The model under review builds one solid part; all positions refer to its coordinate system, in mm. Coordinates: 2 decimals unless noted, no trailing zeros. Write each loop counter-clockwise with the first axis right and the second up, starting at its lowest first coordinate (ties: lowest second). Pieces come first, ordered by that corner, then holes. Notation, with made-up numbers: (16, -11.5) - (47, -11.5) arc R33 ccw to (47, 21.5) - close; hole circle Ø3 at (58, -6). An arc over 180 degrees is marked (long way). Return JSON: item names as keys, results as strings. Group by question number.
(1) We need section B-B on x = 5.5. State the section outline as (y, z) points, then the cut area to 3 significant figures.
(2) We need section A-A on y = -37.5. State the section outline as (x, z) points, then the cut area to 3 significant figures.
(3) For pin 1 Ø6.5 at (x, y) = (-159, -94.5) entering from -Z; pin 2 Ø1.8 at (x, y) = (124, -21) entering from +Z; pin 3 Ø7.5 at (x, z) = (-165, 42.5) entering from +Y, all flat-tipped, find the tip position at first contact; note any pin that passes through.
(4) To check wall thickness, follow L1, parallel to Z at x = -309, y = -73; L2, parallel to Y at x = 258, z = 210; L3, parallel to Y at x = 310.5, z = -38.5. State the ranges of each line that lie inside material, in increasing order. Write a range as from..to.
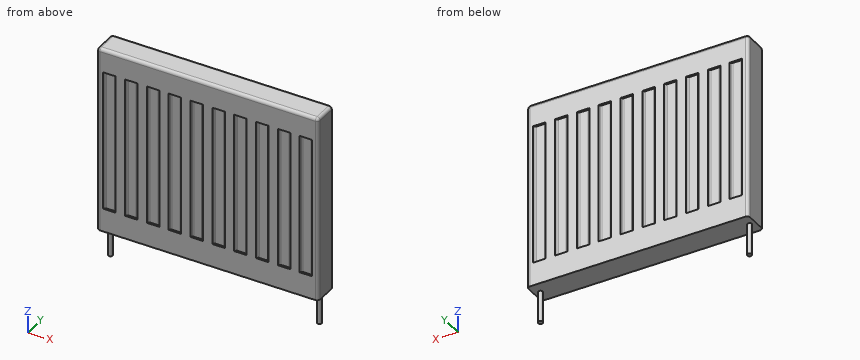
```python
from build123d import *

# Parameters (mm, degrees)
F0_W     = 710
F0_H     = 80
F1_DEPTH = 300
F2_R     = 7.5
F3_DEPTH = 100
F5_DEPTH = 225
F6_R     = 10


with BuildPart() as f1:
    # F0 (on Top) → F1 (new body, symmetric)
    with BuildSketch(Plane.XY):
        with Locations((9.33931, -58.683639)):
            Rectangle(F0_W, F0_H)
    extrude(amount=F1_DEPTH, both=True)

    # F2 (on face) → F3 (join)
    with BuildSketch(Plane(origin=(0, 0, -300), x_dir=(1, 0, 0), z_dir=(0, 0, -1))):
        with Locations((344.33931, 58.683639)):
            Circle(F2_R)
        with Locations((-325.66069, 58.683639)):
            Circle(F2_R)
    extrude(amount=F3_DEPTH)

    # F4 (on Top) → F5 (cut, symmetric)
    with BuildSketch(Plane.XY):
        with BuildLine():
            Line((-285.66069, -18.683639), (-325.66069, -18.683639))
            Line((-325.66069, -18.683639), (-322.124776, -22.897577))
            ThreePointArc((-322.124776, -22.897577), (-320.407645, -24.215178), (-318.294554, -24.683639))
            Line((-318.294554, -24.683639), (-293.026826, -24.683639))
            ThreePointArc((-293.026826, -24.683639), (-290.913735, -24.215178), (-289.196604, -22.897577))
            Line((-289.196604, -22.897577), (-285.66069, -18.683639))
        make_face()
        with BuildLine():
            Line((-215.66069, -18.683639), (-255.66069, -18.683639))
            Line((-255.66069, -18.683639), (-252.124776, -22.897577))
            ThreePointArc((-252.124776, -22.897577), (-250.407645, -24.215178), (-248.294554, -24.683639))
            Line((-248.294554, -24.683639), (-223.026826, -24.683639))
            ThreePointArc((-223.026826, -24.683639), (-220.913735, -24.215178), (-219.196604, -22.897577))
            Line((-219.196604, -22.897577), (-215.66069, -18.683639))
        make_face()
        with BuildLine():
            Line((-145.66069, -18.683639), (-185.66069, -18.683639))
            Line((-185.66069, -18.683639), (-182.124776, -22.897577))
            ThreePointArc((-182.124776, -22.897577), (-180.407645, -24.215178), (-178.294554, -24.683639))
            Line((-178.294554, -24.683639), (-153.026826, -24.683639))
            ThreePointArc((-153.026826, -24.683639), (-150.913735, -24.215178), (-149.196604, -22.897577))
            Line((-149.196604, -22.897577), (-145.66069, -18.683639))
        make_face()
        with BuildLine():
            Line((-75.66069, -18.683639), (-115.66069, -18.683639))
            Line((-115.66069, -18.683639), (-112.124776, -22.897577))
            ThreePointArc((-112.124776, -22.897577), (-110.407645, -24.215178), (-108.294554, -24.683639))
            Line((-108.294554, -24.683639), (-83.026826, -24.683639))
            ThreePointArc((-83.026826, -24.683639), (-80.913735, -24.215178), (-79.196604, -22.897577))
            Line((-79.196604, -22.897577), (-75.66069, -18.683639))
        make_face()
        with BuildLine():
            Line((-5.66069, -18.683639), (-45.66069, -18.683639))
            Line((-45.66069, -18.683639), (-42.124776, -22.897577))
            ThreePointArc((-42.124776, -22.897577), (-40.407645, -24.215178), (-38.294554, -24.683639))
            Line((-38.294554, -24.683639), (-13.026826, -24.683639))
            ThreePointArc((-13.026826, -24.683639), (-10.913735, -24.215178), (-9.196604, -22.897577))
            Line((-9.196604, -22.897577), (-5.66069, -18.683639))
        make_face()
        with BuildLine():
            Line((64.33931, -18.683639), (24.33931, -18.683639))
            Line((24.33931, -18.683639), (27.875224, -22.897577))
            ThreePointArc((27.875224, -22.897577), (29.592355, -24.215178), (31.705446, -24.683639))
            Line((31.705446, -24.683639), (56.973174, -24.683639))
            ThreePointArc((56.973174, -24.683639), (59.086265, -24.215178), (60.803396, -22.897577))
            Line((60.803396, -22.897577), (64.33931, -18.683639))
        make_face()
        with BuildLine():
            Line((134.33931, -18.683639), (94.33931, -18.683639))
            Line((94.33931, -18.683639), (97.875224, -22.897577))
            ThreePointArc((97.875224, -22.897577), (99.592355, -24.215178), (101.705446, -24.683639))
            Line((101.705446, -24.683639), (126.973174, -24.683639))
            ThreePointArc((126.973174, -24.683639), (129.086265, -24.215178), (130.803396, -22.897577))
            Line((130.803396, -22.897577), (134.33931, -18.683639))
        make_face()
        with BuildLine():
            Line((204.33931, -18.683639), (164.33931, -18.683639))
            Line((164.33931, -18.683639), (167.875224, -22.897577))
            ThreePointArc((167.875224, -22.897577), (169.592355, -24.215178), (171.705446, -24.683639))
            Line((171.705446, -24.683639), (196.973174, -24.683639))
            ThreePointArc((196.973174, -24.683639), (199.086265, -24.215178), (200.803396, -22.897577))
            Line((200.803396, -22.897577), (204.33931, -18.683639))
        make_face()
        with BuildLine():
            Line((274.33931, -18.683639), (234.33931, -18.683639))
            Line((234.33931, -18.683639), (237.875224, -22.897577))
            ThreePointArc((237.875224, -22.897577), (239.592355, -24.215178), (241.705446, -24.683639))
            Line((241.705446, -24.683639), (266.973174, -24.683639))
            ThreePointArc((266.973174, -24.683639), (269.086265, -24.215178), (270.803396, -22.897577))
            Line((270.803396, -22.897577), (274.33931, -18.683639))
        make_face()
        with BuildLine():
            Line((344.33931, -18.683639), (304.33931, -18.683639))
            Line((304.33931, -18.683639), (307.875224, -22.897577))
            ThreePointArc((307.875224, -22.897577), (309.592355, -24.215178), (311.705446, -24.683639))
            Line((311.705446, -24.683639), (336.973174, -24.683639))
            ThreePointArc((336.973174, -24.683639), (339.086265, -24.215178), (340.803396, -22.897577))
            Line((340.803396, -22.897577), (344.33931, -18.683639))
        make_face()
        with BuildLine():
            ThreePointArc((-318.294554, -92.683639), (-320.407645, -93.1521), (-322.124776, -94.469701))
            Line((-322.124776, -94.469701), (-325.66069, -98.683639))
            Line((-325.66069, -98.683639), (-285.66069, -98.683639))
            Line((-285.66069, -98.683639), (-289.196604, -94.469701))
            ThreePointArc((-289.196604, -94.469701), (-290.913735, -93.1521), (-293.026826, -92.683639))
            Line((-293.026826, -92.683639), (-318.294554, -92.683639))
        make_face()
        with BuildLine():
            Line((-252.124776, -94.469701), (-255.66069, -98.683639))
            Line((-255.66069, -98.683639), (-215.66069, -98.683639))
            Line((-215.66069, -98.683639), (-219.196604, -94.469701))
            ThreePointArc((-219.196604, -94.469701), (-220.913735, -93.1521), (-223.026826, -92.683639))
            Line((-223.026826, -92.683639), (-248.294554, -92.683639))
            ThreePointArc((-248.294554, -92.683639), (-250.407645, -93.1521), (-252.124776, -94.469701))
        make_face()
        with BuildLine():
            ThreePointArc((200.803396, -94.469701), (199.086265, -93.1521), (196.973174, -92.683639))
            Line((196.973174, -92.683639), (171.705446, -92.683639))
            ThreePointArc((171.705446, -92.683639), (169.592355, -93.1521), (167.875224, -94.469701))
            Line((167.875224, -94.469701), (164.33931, -98.683639))
            Line((164.33931, -98.683639), (204.33931, -98.683639))
            Line((204.33931, -98.683639), (200.803396, -94.469701))
        make_face()
        with BuildLine():
            Line((-112.124776, -94.469701), (-115.66069, -98.683639))
            Line((-115.66069, -98.683639), (-75.66069, -98.683639))
            Line((-75.66069, -98.683639), (-79.196604, -94.469701))
            ThreePointArc((-79.196604, -94.469701), (-80.913735, -93.1521), (-83.026826, -92.683639))
            Line((-83.026826, -92.683639), (-108.294554, -92.683639))
            ThreePointArc((-108.294554, -92.683639), (-110.407645, -93.1521), (-112.124776, -94.469701))
        make_face()
        with BuildLine():
            Line((-145.66069, -98.683639), (-149.196604, -94.469701))
            ThreePointArc((-149.196604, -94.469701), (-150.913735, -93.1521), (-153.026826, -92.683639))
            Line((-153.026826, -92.683639), (-178.294554, -92.683639))
            ThreePointArc((-178.294554, -92.683639), (-180.407645, -93.1521), (-182.124776, -94.469701))
            Line((-182.124776, -94.469701), (-185.66069, -98.683639))
            Line((-185.66069, -98.683639), (-145.66069, -98.683639))
        make_face()
        with BuildLine():
            Line((307.875224, -94.469701), (304.33931, -98.683639))
            Line((304.33931, -98.683639), (344.33931, -98.683639))
            Line((344.33931, -98.683639), (340.803396, -94.469701))
            ThreePointArc((340.803396, -94.469701), (339.086265, -93.1521), (336.973174, -92.683639))
            Line((336.973174, -92.683639), (311.705446, -92.683639))
            ThreePointArc((311.705446, -92.683639), (309.592355, -93.1521), (307.875224, -94.469701))
        make_face()
        with BuildLine():
            Line((-42.124776, -94.469701), (-45.66069, -98.683639))
            Line((-45.66069, -98.683639), (-5.66069, -98.683639))
            Line((-5.66069, -98.683639), (-9.196604, -94.469701))
            ThreePointArc((-9.196604, -94.469701), (-10.913735, -93.1521), (-13.026826, -92.683639))
            Line((-13.026826, -92.683639), (-38.294554, -92.683639))
            ThreePointArc((-38.294554, -92.683639), (-40.407645, -93.1521), (-42.124776, -94.469701))
        make_face()
        with BuildLine():
            Line((64.33931, -98.683639), (60.803396, -94.469701))
            ThreePointArc((60.803396, -94.469701), (59.086265, -93.1521), (56.973174, -92.683639))
            Line((56.973174, -92.683639), (31.705446, -92.683639))
            ThreePointArc((31.705446, -92.683639), (29.592355, -93.1521), (27.875224, -94.469701))
            Line((27.875224, -94.469701), (24.33931, -98.683639))
            Line((24.33931, -98.683639), (64.33931, -98.683639))
        make_face()
        with BuildLine():
            ThreePointArc((270.803396, -94.469701), (269.086265, -93.1521), (266.973174, -92.683639))
            Line((266.973174, -92.683639), (241.705446, -92.683639))
            ThreePointArc((241.705446, -92.683639), (239.592355, -93.1521), (237.875224, -94.469701))
            Line((237.875224, -94.469701), (234.33931, -98.683639))
            Line((234.33931, -98.683639), (274.33931, -98.683639))
            Line((274.33931, -98.683639), (270.803396, -94.469701))
        make_face()
        with BuildLine():
            Line((97.875224, -94.469701), (94.33931, -98.683639))
            Line((94.33931, -98.683639), (134.33931, -98.683639))
            Line((134.33931, -98.683639), (130.803396, -94.469701))
            ThreePointArc((130.803396, -94.469701), (129.086265, -93.1521), (126.973174, -92.683639))
            Line((126.973174, -92.683639), (101.705446, -92.683639))
            ThreePointArc((101.705446, -92.683639), (99.592355, -93.1521), (97.875224, -94.469701))
        make_face()
    extrude(amount=F5_DEPTH, both=True, mode=Mode.SUBTRACT)

    # F6
    f6_edges = [f1.edges().sort_by_distance(p)[0] for p in [
        (-345.66069, -98.683639, 0),
        (-345.66069, -18.683639, 0),
        (364.33931, -98.683639, 0),
        (364.33931, -18.683639, 0),
        (9.33931, -98.683639, 300),
        (9.33931, -18.683639, 300),
        (364.33931, -58.683639, 300),
        (-345.66069, -58.683639, 300),
    ]]
    fillet(f6_edges, radius=F6_R)


solid = f1.part
```
Ans:
{
 "1": {"outline": "(-98.68, -300) - (-18.68, -300) - (-18.68, 290) arc R10 ccw to (-28.68, 300) - (-88.68, 300) arc R10 ccw to (-98.68, 290) - close", "area": "48,000 mm²"},
 "2": {"outline": "(-345.66, -300) - (364.34, -300) - (364.34, 290) arc R10 ccw to (354.34, 300) - (-335.66, 300) arc R10 ccw to (-345.66, 290) - close", "area": "426,000 mm²"},
 "3": {"pin 1": "z = -300", "pin 2": "z = 297.35", "pin 3": "y = -24.68"},
 "4": {"L1": "-300..300", "L2": "-92.68..-24.68", "L3": "-92.83..-24.54"}
}
